For this review, take the finished solid that the model builds, in its own axes (mm). Face numbers are marked on the shaded views. A direction names the side the tool comes from. Coordinates: 2 decimals unless noted, no trailing zeros. Loops run counter-clockwise (first coordinate to the right, second up) from the corner with the lowest first, then second, coordinate; pieces in that order, holes last. Notation, with made-up numbers: (17, -16.75) -> (76, -16.75) arc R6 cw to (76, -8.75) -> close; hole circle Ø7 at (48.25, -29.75). An arc over 180 degrees is marked (long way). One line per item, written item: value.
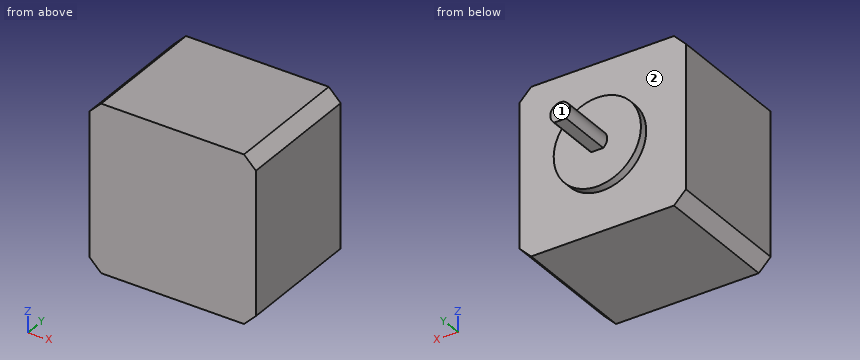
from build123d import *

# Parameters (mm, degrees)
BOSS_EXTRUDE1_DEPTH = 32
SKETCH2_R           = 11
BOSS_EXTRUDE2_DEPTH = 2
BOSS_EXTRUDE3_DEPTH = 14


with BuildPart() as part:
    # Sketch1 → Boss-Extrude1 (new body)
    with BuildSketch(Plane(origin=(0, 0, 0), x_dir=(1, 0, 0), z_dir=(0, 1, 0))):
        Polygon((-18, 21), (-21, 18), (-21, -18), (-18, -21), (18, -21), (21, -18), (21, 18), (18, 21), align=None)
    extrude(amount=BOSS_EXTRUDE1_DEPTH)

    # Sketch2 → Boss-Extrude2 (add)
    with BuildSketch(Plane(origin=(0, 32, 0), x_dir=(1, 0, 0), z_dir=(0, 1, 0))):
        with Locations(Location((0, 0, 0), (0, 0, 270))):
            Circle(SKETCH2_R)
    extrude(amount=BOSS_EXTRUDE2_DEPTH)

    # Sketch3 → Boss-Extrude3 (add)
    with BuildSketch(Plane(origin=(0, 34, 0), x_dir=(1, 0, 0), z_dir=(0, 1, 0))):
        with BuildLine():
            Line((-1.5, 2), (1.5, 2))
            ThreePointArc((1.5, 2), (0, -2.5), (-1.5, 2))
        make_face()
    extrude(amount=BOSS_EXTRUDE3_DEPTH)


solid = part.part
1. Insertion check: pin 1 Ø2.5 at (x, y) = (0, 43.5) entering from -Z; pin 2 Ø6 at (x, z) = (-5.5, 5) entering from +Y. Each pin has a flat end and moves straight along its axis. Give the tip position at first contact, or say it passes through.
Return value:
pin 1: stops at z = -2
pin 2: stops at y = 34
2. Take a section at C-C, the plane z = 6. Give the boundary of the cut face in (x, y), and give its area (3 significant figures).
Return value:
outline: (-21, 0) -> (21, 0) -> (21, 32) -> (9.22, 32) -> (9.22, 34) -> (-9.22, 34) -> (-9.22, 32) -> (-21, 32) -> close
area: 1,380 mm2
3. To check wall thickness, follow probe 1 along Y at (x, z) = (1.5, 15.5); probe 2 along Y at (x, z) = (-1, 7); probe 3 along Z at (x, y) = (-2, 37). State the ranges of each line that lie inside material, in increasing order. Write a range as from..to.
Return value:
probe 1: y = 0..32
probe 2: y = 0..34
probe 3: z = -1.5..1.5
4. Take a section at A-A, the plane z = 0. Give the boundary of the cut face in (x, y), and give its area (3 significant figures).
Return value:
outline: (-21, 0) -> (21, 0) -> (21, 32) -> (11, 32) -> (11, 34) -> (2.5, 34) -> (2.5, 48) -> (-2.5, 48) -> (-2.5, 34) -> (-11, 34) -> (-11, 32) -> (-21, 32) -> close
area: 1,460 mm2
5. Take a section at D-D, the plane x = -8.5. Give the boundary of the cut face in (y, z), and give its area (3 significant figures).
Return value:
outline: (0, -21) -> (32, -21) -> (32, -6.98) -> (34, -6.98) -> (34, 6.98) -> (32, 6.98) -> (32, 21) -> (0, 21) -> close
area: 1,370 mm2
6. Take a section at B-B, the plane x = 0. Give the boundary of the cut face in (y, z), and give its area (3 significant figures).
Return value:
outline: (0, -21) -> (32, -21) -> (32, -11) -> (34, -11) -> (34, -2) -> (48, -2) -> (48, 2.5) -> (34, 2.5) -> (34, 11) -> (32, 11) -> (32, 21) -> (0, 21) -> close
area: 1,450 mm2
7. For the marked faces 1 and 2, list the 3-axis set-ups (+Z, -Z, +X, -X, +Y, -Y) from which the entire face can be reached by the end or side of a thin tool; tool diameter is ignored.
Return value:
face 1: +Z, -Z, +X, -X, +Y
face 2: +Y
